```python
from build123d import *

# Parameters (mm, degrees)
F0_R     = 1.65
F1_DEPTH = 0.5
F2_DEPTH = 1


with BuildPart() as f1:
    # F0 (on Top) → F1 (new body)
    with BuildSketch(Plane.XY):
        with Locations((7.655694, 52.305)):
            Circle(F0_R)
        with BuildLine():
            ThreePointArc((89.305694, 52.305), (87.655694, 53.955), (86.005694, 52.305))
            ThreePointArc((86.005694, 52.305), (87.655694, 50.655), (89.305694, 52.305))
        make_face()
        with BuildLine():
            ThreePointArc((92.655694, 52.305), (91.191228, 55.840534), (87.655694, 57.305))
            Line((87.655694, 57.305), (7.655694, 57.305))
            ThreePointArc((7.655694, 57.305), (4.12016, 55.840534), (2.655694, 52.305))
            Line((2.655694, 52.305), (2.655694, 2.305))
            ThreePointArc((2.655694, 2.305), (4.12016, -1.230534), (7.655694, -2.695))
            Line((7.655694, -2.695), (87.655694, -2.695))
            ThreePointArc((87.655694, -2.695), (91.191228, -1.230534), (92.655694, 2.305))
            Line((92.655694, 2.305), (92.655694, 52.305))
        make_face()
        with Locations((7.655694, 2.305)):
            Circle(F0_R, mode=Mode.SUBTRACT)
        with Locations((14.605, 3.175)):
            Circle(F0_R, mode=Mode.SUBTRACT)
        Polygon((8.679579, 23.260895), (13.055694, 25.697895), (13.055694, 24.38768), (8.653374, 21.845862), (4.251055, 24.38768), (4.251055, 30.07397), (8.679579, 27.636997), (11.745485, 29.36645), (8.653374, 31.069739), (7.710021, 30.571854), (10.068401, 29.183032), (8.810601, 28.50173), (5.299226, 30.571854), (8.679579, 32.484765), (13.055694, 29.942947), (13.055694, 28.763775), (8.653374, 26.221977), (5.56127, 27.95145), (5.56127, 27.165331), (8.679579, 25.462055), (13.055694, 27.872837), (13.055694, 26.562635), (8.653374, 24.047022), (5.56127, 25.802713), (5.56127, 24.990375), align=None, mode=Mode.SUBTRACT)
        with Locations((87.655694, 2.305)):
            Circle(F0_R, mode=Mode.SUBTRACT)
        with Locations((80.645, 6.35)):
            Circle(F0_R, mode=Mode.SUBTRACT)
        with BuildLine():
            Line((19.646068, 43.635763), (75.66532, 43.635763))
            ThreePointArc((75.66532, 43.635763), (79.200854, 42.171297), (80.66532, 38.635763))
            Line((80.66532, 38.635763), (80.66532, 15.974237))
            ThreePointArc((80.66532, 15.974237), (79.200854, 12.438703), (75.66532, 10.974237))
            Line((75.66532, 10.974237), (19.646068, 10.974237))
            ThreePointArc((19.646068, 10.974237), (16.110534, 12.438703), (14.646068, 15.974237))
            Line((14.646068, 15.974237), (14.646068, 38.635763))
            ThreePointArc((14.646068, 38.635763), (16.110534, 42.171297), (19.646068, 43.635763))
        make_face(mode=Mode.SUBTRACT)
        with Locations((7.655694, 52.305)):
            Circle(F0_R, mode=Mode.SUBTRACT)
        with BuildLine():
            ThreePointArc((16.006999, 52.305), (16.191789, 51.887329), (16.255, 51.435))
            ThreePointArc((16.255, 51.435), (14.152671, 49.848211), (13.203001, 52.305))
            ThreePointArc((13.203001, 52.305), (14.605, 53.085), (16.006999, 52.305))
        make_face(mode=Mode.SUBTRACT)
        with Locations((80.645, 48.26)):
            Circle(F0_R, mode=Mode.SUBTRACT)
        with BuildLine():
            ThreePointArc((89.305694, 52.305), (87.655694, 50.655), (86.005694, 52.305))
            ThreePointArc((86.005694, 52.305), (87.655694, 53.955), (89.305694, 52.305))
        make_face(mode=Mode.SUBTRACT)
        Polygon((13.055694, 24.38768), (13.055694, 25.697895), (8.679579, 23.260895), (5.56127, 24.990375), (5.56127, 25.802713), (8.653374, 24.047022), (13.055694, 26.562635), (13.055694, 27.872837), (8.679579, 25.462055), (5.56127, 27.165331), (5.56127, 27.95145), (8.653374, 26.221977), (13.055694, 28.763775), (13.055694, 29.942947), (8.679579, 32.484765), (5.299226, 30.571854), (8.810601, 28.50173), (10.068401, 29.183032), (7.710021, 30.571854), (8.653374, 31.069739), (11.745485, 29.36645), (8.679579, 27.636997), (4.251055, 30.07397), (4.251055, 24.38768), (8.653374, 21.845862), align=None)
    extrude(amount=F1_DEPTH)

    # F0 (on Top) → F2 (join)
    with BuildSketch(Plane.XY):
        Polygon((13.055694, 24.38768), (13.055694, 25.697895), (8.679579, 23.260895), (5.56127, 24.990375), (5.56127, 25.802713), (8.653374, 24.047022), (13.055694, 26.562635), (13.055694, 27.872837), (8.679579, 25.462055), (5.56127, 27.165331), (5.56127, 27.95145), (8.653374, 26.221977), (13.055694, 28.763775), (13.055694, 29.942947), (8.679579, 32.484765), (5.299226, 30.571854), (8.810601, 28.50173), (10.068401, 29.183032), (7.710021, 30.571854), (8.653374, 31.069739), (11.745485, 29.36645), (8.679579, 27.636997), (4.251055, 30.07397), (4.251055, 24.38768), (8.653374, 21.845862), align=None)
    extrude(amount=F2_DEPTH)


solid = f1.part
```
Here's how the part is built. I have some questions about the finished solid (model axes, mm). A direction names the side the tool comes from. Round coordinates to 2 decimals unless told otherwise and drop trailing zeros. Loops run counter-clockwise (first coordinate to the right, second up) from the corner with the lowest first, then second, coordinate; pieces in that order, holes last.
1. Thinking about a two-plate mould opening in Y: for faces 4 (the face through (9, 27, 1)), 5 (the face through (10.824, 23.099, 0.746)), 6 (the face through (10.898, 24.496, 0.746)), which applies, released by +Y, released by -Y, zero draft, split by the parting line, or undercut?
Answers:
face 4: zero draft
face 5: released by -Y
face 6: undercut
2. Suppose I cut it at A-A, the plane y = 6.35. Please give me the cut outline in (x, z) (3 decimals), and give its area (4 significant figures).
Answers:
outline: (2.656, 0) - (78.995, 0) - (78.995, 0.5) - (2.656, 0.5) - close; (82.295, 0) - (92.656, 0) - (92.656, 0.5) - (82.295, 0.5) - close
area: 43.35 mm2
3. If I drill on probe 1 along X at (y, z) = (35, 0.15); probe 2 along X at (y, z) = (29, 0.6); probe 3 along Y at (x, z) = (71.5, 0.1) (3 decimals), over which ranges is the centre line in solid material (lowest first)?
Answers:
probe 1: x = 2.66 to 14.65, 80.67 to 92.66
probe 2: x = 4.25 to 6.2, 7.97 to 9.73, 11.1 to 13.06
probe 3: y = -2.695 to 10.974, 43.636 to 57.305
4. Suppose I cut it at D-D, the plane x = 84.5. Please give me the cut outline in (y, z) (3 decimals).
Answers:
outline: (-2.695, 0) - (57.305, 0) - (57.305, 0.5) - (-2.695, 0.5) - close
5. Suppose I cut it at B-B, the plane x = 34. Please give me the cut outline in (y, z) (3 decimals).
Answers:
outline: (-2.695, 0) - (10.974, 0) - (10.974, 0.5) - (-2.695, 0.5) - close; (43.636, 0) - (57.305, 0) - (57.305, 0.5) - (43.636, 0.5) - close
6. Will these pins go through, and if not, where does the flat tip stop? pin 1 (4.5 mm diameter, centred on x = 7.66, y = 2.31, fed in from +Z); pin 2 (2.5 mm diameter, centred on x = 7.66, y = 52.3, fed in from -Z); pin 3 (0.6 mm diameter, centred on y = 27.5, z = 1, fed in from +X).
Answers:
pin 1: stops at z = 0.5
pin 2: passes through
pin 3: stops at x = 13.06
7. For faces 1 (the face through (6.421, 23.135, 0.746)), 2 (the face through (10.824, 27.475, 0.746)), 3 (the face through (16.15, 12.4, 0.25)), which set-ups out of +Z, -Z, +X, -X, +Y, -Y let a thin tool reach every point of the face, with its end or its side?
Answers:
face 1: +Z, -X, -Y
face 2: +Z
face 3: +Z, -Z
8. Suppose I cut it at C-C, the plane z = 0.75. Please give me the cut outline in (x, y), and give its area (3 significant figures).
Answers:
outline: (4.25, 24.39) - (8.65, 21.85) - (13.06, 24.39) - (13.06, 25.7) - (8.68, 23.26) - (5.56, 24.99) - (5.56, 25.8) - (8.65, 24.05) - (13.06, 26.56) - (13.06, 27.87) - (8.68, 25.46) - (5.56, 27.17) - (5.56, 27.95) - (8.65, 26.22) - (13.06, 28.76) - (13.06, 29.94) - (8.68, 32.48) - (5.3, 30.57) - (8.81, 28.5) - (10.07, 29.18) - (7.71, 30.57) - (8.65, 31.07) - (11.75, 29.37) - (8.68, 27.64) - (4.25, 30.07) - close
area: 50.6 mm2
